from build123d import *

# Parameters (mm, degrees)
SKETCH1_R           = 25
BOSS_EXTRUDE1_DEPTH = 3
SKETCH2_R           = 1.75
CUT_EXTRUDE1_DEPTH  = 3
CIRPATTERN1_COUNT   = 8
CUT_EXTRUDE2_DEPTH  = 10
FILLET1_R           = 1


with BuildPart() as part:
    # Sketch1 → Boss-Extrude1 (new body)
    with BuildSketch(Plane.XY):
        Circle(SKETCH1_R)
    extrude(amount=BOSS_EXTRUDE1_DEPTH)

    # Sketch2 → Cut-Extrude1 (cut)
    with BuildSketch(Plane.XY.offset(3)):
        with Locations((0, 20)):
            Circle(SKETCH2_R)
    cut_extrude1 = extrude(amount=-CUT_EXTRUDE1_DEPTH, mode=Mode.SUBTRACT)

    # CirPattern1: Cut-Extrude1 ×8 about axis
    cirpattern1_axis = Axis((0, 0, 0), (0, 0, 1))
    for i in range(1, CIRPATTERN1_COUNT):
        add(cut_extrude1.rotate(cirpattern1_axis, i * 360 / CIRPATTERN1_COUNT), mode=Mode.SUBTRACT)

    # Sketch3 → Cut-Extrude2 (cut)
    with BuildSketch(Plane.XY.offset(3)):
        with BuildLine():
            Line((-2.5, 14.790199458), (-2.5, -14.790199458))
            ThreePointArc((-2.5, -14.790199458), (-15, 0), (-2.5, 14.790199458))
        make_face()
        with BuildLine():
            Line((2.5, 14.790199458), (2.5, -14.790199458))
            ThreePointArc((2.5, -14.790199458), (15, 0), (2.5, 14.790199458))
        make_face()
    extrude(amount=-CUT_EXTRUDE2_DEPTH, mode=Mode.SUBTRACT)

    # Fillet1
    fillet1_edges = [part.edges().sort_by_distance(p)[0] for p in [
        (-2.5, -14.790199458, 1.5),
        (-2.5, 14.790199458, 1.5),
        (2.5, 14.790199458, 1.5),
        (2.5, -14.790199458, 1.5),
    ]]
    fillet(fillet1_edges, radius=FILLET1_R)


solid = part.part
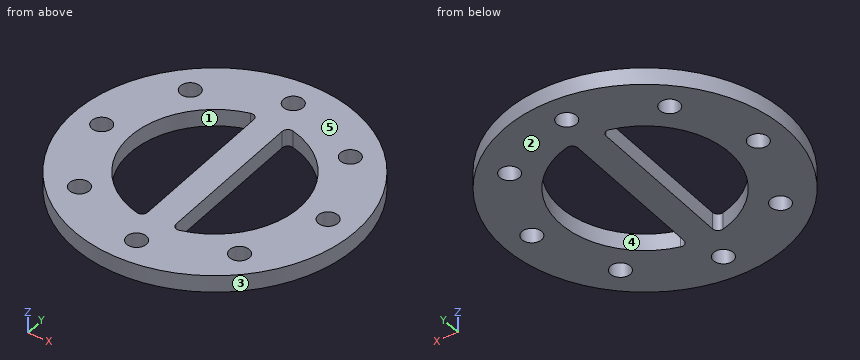
Can you work these out from the model? Positions are in its coordinate system, mm. Face numbers are marked on the shaded views. A direction names the side the tool comes from. Give positions to 0.01 mm unless a question says otherwise; leave off trailing zeros. Order: outer loops, then holes, each group sorted by start corner. A loop starts at its lowest first (then second) coordinate and runs counter-clockwise, first axis right, second up. Notation, with made-up numbers: M 1,82.5 L 58,82.5 A23 cw 58,95.5 Z; hole C 31,9.5 d5. An arc over 180 degrees is marked long. Use one line per item in the form item = value.
Item 1: For the marked faces 4 and 5, which set-ups out of +Z, -Z, +X, -X, +Y, -Y let a thin tool reach every point of the face, with its end or its side?
Values follow:
face_4 = +Z, -Z
face_5 = +Z, +X, -X, +Y, -Y
Item 2: If we section it at D-D, the plane z = 1.65: Count the separate pieces of the cut face and the enclosed holes in it, and give its area (3 significant figures).
Values follow:
separate_pieces = 1
enclosed_holes = 10
area = 1,330 mm^2
Item 3: Thinking about a two-plate mould opening in Y: for the marked faces 1, 2 and 3, which applies, pulls with the +Y half, pulls with the -Y half, needs draft (parallel to the pull), parting line crosses it, or undercut?
Values follow:
face_1 = undercut
face_2 = needs draft
face_3 = parting line crosses it
Item 4: If I drill on line 1 along Y through (x, z) = (-20, 1.85); line 2 along Y through (x, z) = (0, 1.9); line 3 along X through (y, z) = (-9, 1.3), over which ranges is the centre line in solid material (lowest first)? Write a range as [from, to].
Values follow:
line_1 = [-15, -1.75], [1.75, 15]
line_2 = [-25, -21.75], [-18.25, 18.25], [21.75, 25]
line_3 = [-23.32, -12], [-2.5, 2.5], [12, 23.32]
Item 5: If we section it at A-A, the plane y = -20: Write out the boundary of the cut face in (x, z).
Values follow:
outline = M -15,0 L -1.75,0 L -1.75,3 L -15,3 Z; M 1.75,0 L 15,0 L 15,3 L 1.75,3 Z
Item 6: If we section it at C-C, the plane y = 0: Write out the boundary of the cut face in (x, z).
Values follow:
outline = M -25,0 L -21.75,0 L -21.75,3 L -25,3 Z; M -18.25,0 L -15,0 L -15,3 L -18.25,3 Z; M -2.5,0 L 2.5,0 L 2.5,3 L -2.5,3 Z; M 15,0 L 18.25,0 L 18.25,3 L 15,3 Z; M 21.75,0 L 25,0 L 25,3 L 21.75,3 Z
Item 7: If we section it at B-B, the plane x = 13.5: Write out the boundary of the cut face in (y, z), and give its area (3 significant figures).
Values follow:
outline = M -21.04,0 L -15.77,0 L -15.77,3 L -21.04,3 Z; M -12.51,0 L -6.54,0 L -6.54,3 L -12.51,3 Z; M 6.54,0 L 12.51,0 L 12.51,3 L 6.54,3 Z; M 15.77,0 L 21.04,0 L 21.04,3 L 15.77,3 Z
area = 67.5 mm^2
Item 8: Will this pin go through, and if not, where does the flat tip stop? pin 1 Ø0.9 at (y, z) = (-2, 1.5) entering from -X.
Values follow:
pin_1 = -24.95
